```python
from build123d import *

# Parameters (mm, degrees)
SKETCH1_R           = 1.61
BOSS_EXTRUDE1_DEPTH = 9.62
CUT_EXTRUDE1_REACH  = 23.691
SKETCH2_W           = 2.28
SKETCH2_H           = 19.007620098
SKETCH3_W           = 11.260460121
SKETCH3_H           = 2.28
CUT_EXTRUDE2_DEPTH  = 3.04


with BuildPart() as part:
    # Sketch1 → Boss-Extrude1 (new body)
    with BuildSketch(Plane.XY):
        with BuildLine():
            Line((0, 0), (5.140631262, 3.208973392))
            ThreePointArc((5.140631262, 3.208973392), (5.914482507, 3.089800479), (5.911583106, 2.306832072))
            Line((5.911583106, 2.306832072), (1.273331069, -3.04))
            Line((1.273331069, -3.04), (-9.656668931, -3.04))
            Line((-9.656668931, -3.04), (-17.168479282, -11.699380338))
            ThreePointArc((-17.168479282, -11.699380338), (-20.147653582, -13.029479565), (-23.08154503, -11.60227095))
            Line((-23.08154503, -11.60227095), (-24.370177587, -10.154805065))
            ThreePointArc((-24.370177587, -10.154805065), (-25.319176443, -9.441943032), (-26.47036432, -9.152914355))
            Line((-26.47036432, -9.152914355), (-31.285658795, -8.927140459))
            ThreePointArc((-31.285658795, -8.927140459), (-32.860887009, -6.762353106), (-30.871741613, -4.970441053))
            Line((-30.871741613, -4.970441053), (-25.191741613, -4.970441053))
            Line((-25.191741613, -4.970441053), (-20.88, 0))
            Line((-20.88, 0), (0, 0))
        make_face()
        with Locations((-20.08426993, -9.17)):
            Circle(SKETCH1_R, mode=Mode.SUBTRACT)
    extrude(amount=BOSS_EXTRUDE1_DEPTH)

    # Cut-Extrude1: up to this face of the body (flat: up to its plane)
    cut_extrude1_end = Plane(part.part.faces().sort_by_distance((-4.191668931, -3.04, 4.81))[0])
    # Sketch2 → Cut-Extrude1 (cut, up to the picked face)
    with BuildSketch(Plane(origin=(-4.005407565, 3.474597584, 0), x_dir=(0, 0, -1), z_dir=(0.755386178, -0.65527988, 0)), mode=Mode.PRIVATE) as cut_extrude1_sk1:
        with Locations((-4.81, -18.128004893)):
            Rectangle(SKETCH2_W, SKETCH2_H)
    cut_extrude1_tool1 = split(extrude(cut_extrude1_sk1.sketch, amount=-CUT_EXTRUDE1_REACH, mode=Mode.PRIVATE), bisect_by=cut_extrude1_end, keep=Keep.BOTH, mode=Mode.PRIVATE)
    add(cut_extrude1_tool1.solids().sort_by_distance((-15.884324, -10.219047, 4.81))[0], mode=Mode.SUBTRACT)

    # Sketch3 → Cut-Extrude2 (cut)
    with BuildSketch(Plane.XZ.offset(3.04)):
        with Locations((-17.886898992, 4.81)):
            Rectangle(SKETCH3_W, SKETCH3_H)
    extrude(amount=-CUT_EXTRUDE2_DEPTH, mode=Mode.SUBTRACT)


solid = part.part
```
Design review of the part built by this model. Coordinates are the model's own, in mm. A direction names the side the tool comes from. Coordinates: 2 decimals unless noted, no trailing zeros. Loops run counter-clockwise (first coordinate to the right, second up) from the corner with the lowest first, then second, coordinate; pieces in that order, holes last. Notation, with made-up numbers: M 28,-9 L 80,-9 A18 ccw 80,15 Z; hole C 1,49.25 d8. An arc over 180 degrees is marked long. One line per question, with ' | ' between items.
(1) Draft analysis for pull direction X (two halves, no side actions). For faces 1 (the face through (-12.257, -2, 5)), 2 (the face through (-16, -5, 9.62)), 3 (the face through (-21.4, -10.1, 1.8)), state which applies: released by +X, released by -X, zero draft, split by the parting line, or undercut.
Filled in:
face 1: released by -X | face 2: zero draft | face 3: undercut
(2) Wall thickness on probe 1 along Z at (x, y) = (-21, -11); probe 2 along Y at (x, z) = (-7.5, 1.25); probe 3 along Y at (x, z) = (-29, 8): over which ranges is each line inside the solid? List them lowest first.
Filled in:
probe 1: z = 0 to 3.67, 5.95 to 9.62 | probe 2: y = -3.04 to 0 | probe 3: y = -9.03 to -4.97
(3) We need section B-B (x = -27). Give the boundary of the cut face in (y, z), and give its area (3 significant figures).
Filled in:
outline: M -9.13,0 L -4.97,0 L -4.97,3.67 L -9.13,3.67 Z; M -9.13,5.95 L -4.97,5.95 L -4.97,9.62 L -9.13,9.62 Z | area: 30.5 mm^2
(4) We need section C-C (y = -2.5). Give the boundary of the cut face in (x, z).
Filled in:
outline: M -23.05,0 L 1.74,0 L 1.74,9.62 L -23.05,9.62 L -23.05,5.95 L -12.26,5.95 L -12.26,3.67 L -23.05,3.67 Z
(5) We need section A-A (z = 8). Give the boundary of the cut face in (x, y).
Filled in:
outline: M -31.29,-8.93 L -26.47,-9.15 A3 cw -24.37,-10.15 L -23.08,-11.6 A3.86 ccw -17.17,-11.7 L -9.66,-3.04 L 1.27,-3.04 L 5.91,2.31 A0.6 ccw 5.14,3.21 L 0,0 L -20.88,0 L -25.19,-4.97 L -30.87,-4.97 A2 ccw Z; hole C -20.08,-9.17 d3.22
(6) Machinability: for faces 4 (the face through (-11, 0, 5)), 5 (the face through (-32.865, -6.803, 1.809)), which of the approach directions +Z, -Z, +X, -X, +Y, -Y give a long, thin tool a straight path to every point of the face, cutting with its end or side? Answer none if there is none.
Filled in:
face 4: +Z, -Z, -X, +Y | face 5: +Z, -Z, -X
(7) For pin 1 Ø5 at (x, y) = (-20.08, -9.17) entering from -Z; pin 2 Ø1.9 at (x, y) = (-20.08, -9.17) entering from -Z; pin 3 Ø1.5 at (y, z) = (-10, 8) entering from +X; pin 4 Ø4 at (x, z) = (-2, 4) entering from -Y, all flat-tipped, find the tip position at first contact; note any pin that passes through.
Filled in:
pin 1: stops at z = 0 | pin 2: passes through | pin 3: stops at x = -15.04 | pin 4: stops at y = -3.04
(8) We need section D-D (z = 5). Give the boundary of the cut face in (x, y).
Filled in:
outline: M -12.26,-3.04 L 1.27,-3.04 L 5.91,2.31 A0.6 ccw 5.14,3.21 L 0,0 L -12.26,0 Z
